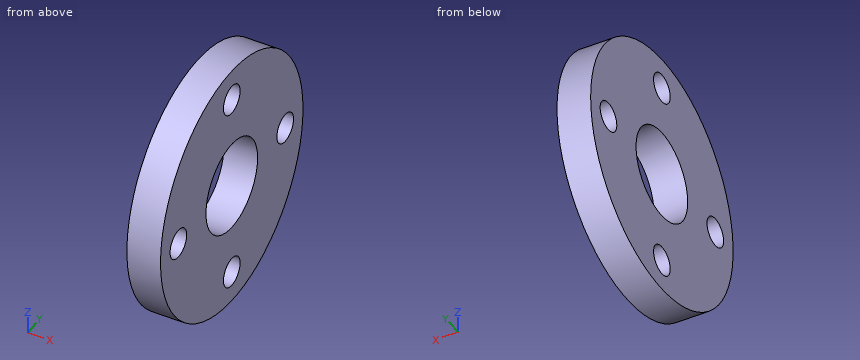
Autodesk Inventor part; units mm, degrees
ref_plane "YZ Plane" through (0, 0, 0) normal (1, 0, 0) x (0, 1, 0)
ref_plane "XZ Plane" through (0, 0, 0) normal (0, 1, 0) x (-1, 0, 0)
ref_plane "XY Plane" through (0, 0, 0) normal (0, 0, 1) x (1, 0, 0)
sketch "Schizzo1" plane through (0, 0, 0) normal (0, 0, 1) x (1, 0, 0)
  line L0 (0, 0) -> (22.1221, 0) construction
  line L1 (0, 0) -> (0, 21.75) construction
  line L2 (0, 60) -> (16, 60)
  line L3 (16, 60) -> (16, 21.75)
  line L4 (16, 21.75) -> (0, 21.75)
  line L5 (0, 21.75) -> (0, 60)
  dimension "d0" = 16
  dimension "d1" = 38.25
  dimension "d2" = 120
revolve "Rivoluzione1" add sketch "Schizzo1" angle 360 about axis through (0, 0, 0) along (1, 0, 0)
sketch "Schizzo2" plane through (0, 0, 0) normal (1, 0, 0) x (0, 1, 0)
  circle A0 centre (0, 0) radius 45
  circle A1 centre (45, 0) radius 7
  dimension "d4" = 90
  dimension "d5" = 14
extrude "Estrusione1" cut sketch "Schizzo2" along normal through all contours A0 A1 | A0 A1 picked at (42.7183, -1.3528) picked at (47.059, -1.8371)
pattern_circular "Serie circolare1" count 4 over 360 about axis through (8, 0, 0) along (1, 0, 0) of "Estrusione1"
properties part number "06-01-2023 flangia piccola"
Could you check a few things on this model? Use its own coordinates, in mm. Coordinates: 2 decimals unless noted, no trailing zeros. Order: outer loops, then holes, each group sorted by start corner. A loop starts at its lowest first (then second) coordinate and runs counter-clockwise, first axis right, second up. Notation, with made-up numbers: (29.5, 68.25) -> (38.5, 68.25) arc R31 ccw to (38.5, 95.25) -> close; hole circle Ø8 at (-19.5, -30.75). An arc over 180 degrees is marked (long way). One line per question, with ' | ' between items.
Q1. Imagine slicing it at D-D on y = 41. Please give me the cut outline in (x, z).
Return value:
outline: (0, -43.81) -> (16, -43.81) -> (16, -5.74) -> (0, -5.74) -> close; (0, 5.74) -> (16, 5.74) -> (16, 43.81) -> (0, 43.81) -> close
Q2. I'm going to push flat-ended pins straight in: P1, Ø5, axis at x = 11.5, z = -16.5, coming from the +Y side; P2, Ø1.5, axis at x = 11, y = -7.5, coming from the +Z side; P3, Ø2, axis at x = 5.5, z = -26, coming from the +Y side; P4, Ø18, axis at y = 0, z = -45, coming from the -X side. Where does each tip first touch, or does it pass through?
Return value:
P1: y = 58.34 | P2: z = 59.62 | P3: y = 54.54 | P4: x = 0
Q3. Imagine slicing it at C-C on x = 4.25. Please give me the cut outline in (y, z).
Return value:
outline: circle Ø120 at (0, 0); hole circle Ø14 at (-45, 0); hole circle Ø43.5 at (0, 0); hole circle Ø14 at (0, -45); hole circle Ø14 at (0, 45); hole circle Ø14 at (45, 0)
Q4. Imagine slicing it at A-A on y = 0. Please give me the cut outline in (x, z).
Return value:
outline: (0, -60) -> (16, -60) -> (16, -52) -> (0, -52) -> close; (0, -38) -> (16, -38) -> (16, -21.75) -> (0, -21.75) -> close; (0, 21.75) -> (16, 21.75) -> (16, 38) -> (0, 38) -> close; (0, 52) -> (16, 52) -> (16, 60) -> (0, 60) -> close
Q5. If I drill on L1, parallel to Z at x = 8.75, y = 0; L2, parallel to Z at x = 10.25, y = -2.5; L3, parallel to Y at x = 11.75, z = -5.5, over which ranges is the centre line in solid material (lowest first)?
Return value:
L1: -60 to -52, -38 to -21.75, 21.75 to 38, 52 to 60 | L2: -59.95 to -51.54, -38.46 to -21.61, 21.61 to 38.46, 51.54 to 59.95 | L3: -59.75 to -49.33, -40.67 to -21.04, 21.04 to 40.67, 49.33 to 59.75
